Here's how the part is built. I have some questions about the finished solid (model axes, mm). Coordinates: 2 decimals unless noted, no trailing zeros. Loops run counter-clockwise (first coordinate to the right, second up) from the corner with the lowest first, then second, coordinate; pieces in that order, holes last. Notation, with made-up numbers: (-38.5, 61) -> (-32.5, 61) arc R34 cw to (-32.5, 95) -> close; hole circle Ø10 at (62, -10.75). An arc over 180 degrees is marked (long way). Answer as a JSON object with one key per item and string values. Group by question number.
1) I want a section at D-D (y = -22.5). Write out the boundary of the cut face in (x, z).
2) I want a section at B-B (x = 24). Write out the boundary of the cut face in (y, z).
3) I'm going to push flat-ended pins straight in: pin 1 (1.5 mm diameter, centred on x = 10, y = -16, fed in from -Z); pin 2 (1 mm diameter, centred on x = 44.5, y = -3.5, fed in from -Z); pin 3 (11.5 mm diameter, centred on x = 29.94, y = -9.54, fed in from +Z). Where does each tip first touch, or does it pass through?
4) If we mould it in two halves opening along Y, with no side actions, what happens to faces 1 (the flat face through (61.127, -12, 26)), 2 (the flat face through (30, -25, 25)), 3 (the cylindrical face through (29.532, -19.114, 25.955))? For each: +Y half, -Y half, draft (parallel to the pull), parting line (faces both ways), or undercut.
5) I want a section at C-C (z = 36). Write out the boundary of the cut face in (x, y), then the cut area to 3 significant figures.
6) I want a section at A-A (y = -16.5). Write out the boundary of the cut face in (x, z), then the cut area to 3 significant figures.
7) I need wall thicknesses on probe 1 along X at (y, z) = (-9.5, 5.5); probe 2 along Y at (x, z) = (35, 20); probe 3 along Y at (x, z) = (32.5, 28). Which ranges of each line are inside material? Lowest first, please. Write a range as [from, to].
```python
from build123d import *

# Parameters (mm, degrees)
F1_DEPTH = 25
F2_R     = 9.584307
F3_DEPTH = 60


with BuildPart() as f1:
    # F0 (on Front) → F1 (new body)
    with BuildSketch(Plane.XZ):
        Polygon((0, 50.165702), (0, 0), (61.127122, 3.314364), (61.127122, 50.165702), align=None)
    extrude(amount=F1_DEPTH)

    # F2 (on face) → F3 (cut)
    with BuildSketch(Plane.XY.offset(50.165702)):
        with Locations((29.940704, -9.538786)):
            Circle(F2_R)
    extrude(amount=-F3_DEPTH, mode=Mode.SUBTRACT)


solid = f1.part
```
Determined:
{
 "1": {"outline": "(0, 0) -> (61.13, 3.31) -> (61.13, 50.17) -> (0, 50.17) -> close"},
 "2": {"outline": "(-25, 1.3) -> (-17.06, 1.3) -> (-17.06, 50.17) -> (-25, 50.17) -> close; (-2.02, 1.3) -> (0, 1.3) -> (0, 50.17) -> (-2.02, 50.17) -> close"},
 "3": {"pin 1": "z = 0.5", "pin 2": "z = 2.39", "pin 3": "through"},
 "4": {"face 1": "draft", "face 2": "-Y half", "face 3": "undercut"},
 "5": {"outline": "(0, -25) -> (61.13, -25) -> (61.13, 0) -> (30.87, 0) arc R9.58 cw (long way) to (29.01, 0) -> (0, 0) -> close", "area": "1,240 mm^2"},
 "6": {"outline": "(0, 0) -> (23.35, 1.27) -> (23.35, 50.17) -> (0, 50.17) -> close; (36.53, 1.98) -> (61.13, 3.31) -> (61.13, 50.17) -> (36.53, 50.17) -> close", "area": "2,330 mm^2"},
 "7": {"probe 1": "[0, 20.36], [39.52, 61.13]", "probe 2": "[-25, -17.68], [-1.4, 0]", "probe 3": "[-25, -18.78], [-0.3, 0]"}
}
